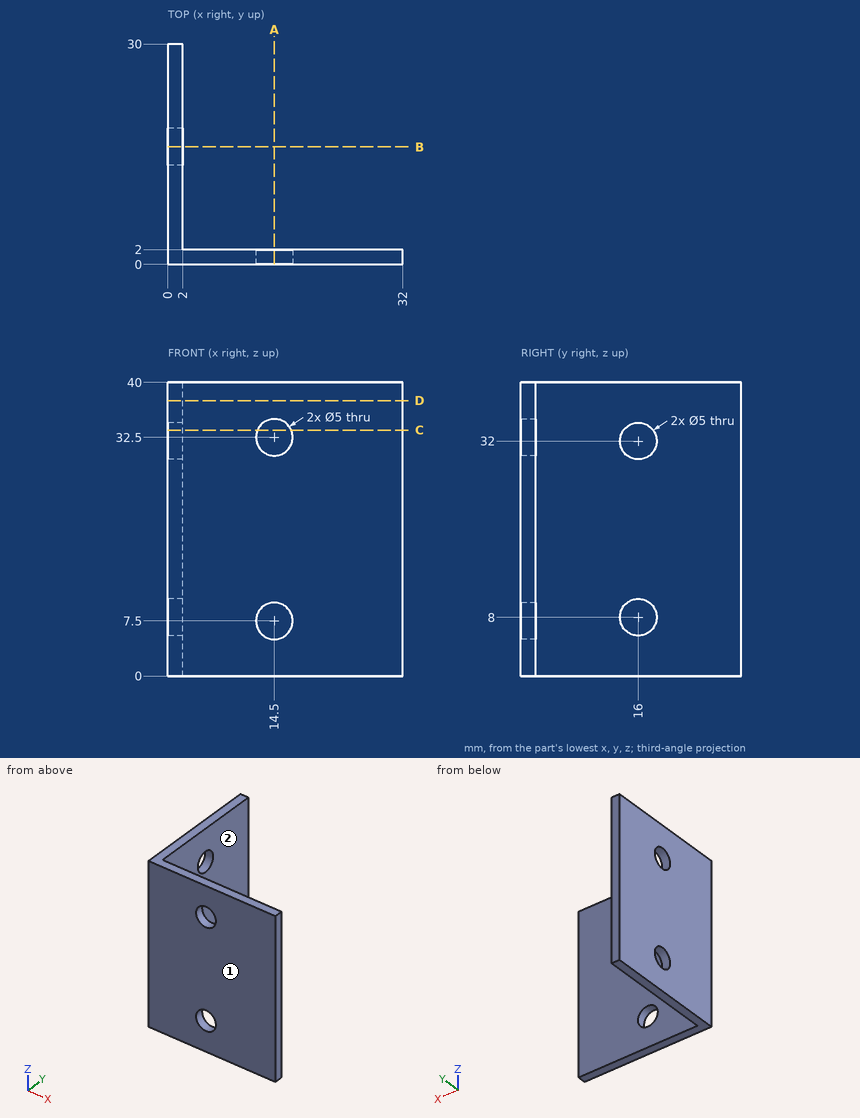
The figure shows three views and two pictorial views of one solid part (mm, origin at its lowest corner). Answer the questions. A direction names the side the tool comes from. Round coordinates to 2 decimals unless told otherwise and drop trailing zeros. Write each loop counter-clockwise with the first axis right and the second up, starting at its lowest first coordinate (ties: lowest second). Pieces come first, ordered by that corner, then holes. Notation, with made-up numbers: (-40, 56.25) - (3, 56.25) arc R17 ccw to (3, 61.25) - close; hole circle Ø8 at (68, 62.25). An arc over 180 degrees is marked (long way). Use one line per item in the form item = value. Start each with the question number.
Item 1: A cutting plane is placed at B-B (y = 16). Write down the section's boundary in (x, z), plus the area to 3 significant figures.
Item 2: Flat-ended cylindrical pins translate along their axes: pin 1 Ø3 at (y, z) = (16, 8) entering from +X; pin 2 Ø2 at (y, z) = (4, 7.5) entering from +X; pin 3 Ø3 at (x, z) = (13.5, 33.5) entering from +Y. Find the tip coordinate at first contact, or state that the pin passes through.
Item 3: A cutting plane is placed at D-D (z = 37.5). Write down the section's boundary in (x, y).
Item 4: A cutting plane is placed at A-A (x = 14.5). Write down the section's boundary in (y, z), plus the area to 3 significant figures.
Item 5: A tool of negligible diameter and unlimited length cuts with its end or side. For the marked faces 1 and 2, from which of +Z, -Z, +X, -X, +Y, -Y can it reach the whole face along a straight path? Write none if from no direction.
Item 6: A cutting plane is placed at C-C (z = 33.5). Write down the section's boundary in (x, y).
Item 7: Find the intervals of material crossed by line 1 (Z direction, x = 14.5, y = 0.65); line 2 (X direction, y = 0.4, z = 32.5); line 3 (X direction, y = 3.75, z = 22.5), in increasing order. Write a range as [from, to].
The answers:
q1.outline = (0, 0) - (2, 0) - (2, 5.5) - (0, 5.5) - close; (0, 10.5) - (2, 10.5) - (2, 29.5) - (0, 29.5) - close; (0, 34.5) - (2, 34.5) - (2, 40) - (0, 40) - close
q1.area = 60.0 mm^2
q2.pin_1 = through
q2.pin_2 = 2
q2.pin_3 = 2
q3.outline = (0, 0) - (32, 0) - (32, 2) - (2, 2) - (2, 30) - (0, 30) - close
q4.outline = (0, 0) - (2, 0) - (2, 5) - (0, 5) - close; (0, 10) - (2, 10) - (2, 30) - (0, 30) - close; (0, 35) - (2, 35) - (2, 40) - (0, 40) - close
q4.area = 60.0 mm^2
q5.face_1 = +Z, -Z, +X, -X, -Y
q5.face_2 = +Z, -Z, +X, +Y
q6.outline = (0, 0) - (12.21, 0) - (12.21, 2) - (2, 2) - (2, 14) - (0, 14) - close; (0, 18) - (2, 18) - (2, 30) - (0, 30) - close; (16.79, 0) - (32, 0) - (32, 2) - (16.79, 2) - close
q7.line_1 = [0, 5], [10, 30], [35, 40]
q7.line_2 = [0, 12], [17, 32]
q7.line_3 = [0, 2]
